Autodesk Inventor part; units mm, degrees
ref_plane "YZ Plane" through (0, 0, 0) normal (1, 0, 0) x (0, 1, 0)
ref_plane "XZ Plane" through (0, 0, 0) normal (0, 1, 0) x (-1, 0, 0)
ref_plane "XY Plane" through (0, 0, 0) normal (0, 0, 1) x (1, 0, 0)
sketch "Esquisse1" plane through (0, 0, 0) normal (0, 1, 0) x (-1, 0, 0)
  circle A0 centre (0, 0) radius 15
  circle A1 centre (0, 0) radius 8
  dimension "d0" = 30
  dimension "d1" = 16
extrude "Extrusion1" add sketch "Esquisse1" along normal blind 5
sketch "Esquisse2" plane through (0, 5, 0) normal (0, 1, 0) x (1, 0, 0)
  circle A0 centre (0, 0) radius 15
  point P0 (-12, 0)
  point P1 (6, -10.3923)
  point P2 (6, 10.3923)
  dimension "d4" = 12
  dimension "d7" = 360
hole "Perçage1" at (-12, 5, 0) at (6, 5, 10.3923) at (6, 5, -10.3923) direction (0, -1, 0) diameter 3 depth 8 tip angle 118
sketch "Esquisse3" plane through (0, 5, 0) normal (0, 1, 0) x (1, 0, 0)
  circle A0 centre (61.032, 0) radius 11
  circle A1 centre (61.032, 0) radius 15
  point P0 (0, 0)
  dimension "d16" = 61.032
  dimension "d17" = 22
  dimension "d18" = 30
extrude "Extrusion2" add sketch "Esquisse3" against normal blind 14
sketch "Esquisse4" plane through (0, 5, 0) normal (0, 1, 0) x (1, 0, 0)
  circle A0 centre (0, 0) radius 8
  line L0 (8, 0) -> (48.6, 0)
  line L1 (48.6, 0) -> (48.6, 2.5)
  line L2 (48.6, 2.5) -> (8, 2.5)
  line L3 (8, 2.5) -> (8, 0)
  line L4 (8, 0) -> (48.6, 0)
  line L5 (48.6, 0) -> (48.6, -2.5)
  line L6 (48.6, -2.5) -> (8, -2.5)
  line L7 (8, -2.5) -> (8, 0)
  dimension "d21" = 2.5
  dimension "d22" = 2.5
  dimension "d23" = 40.6
extrude "Extrusion3" add sketch "Esquisse4" against normal blind 5 contours L3 L2 L1 L0 | L0 L5 L6 L7
properties part number "BarreCodeuseV2"
The model under review builds one solid part; all positions refer to its coordinate system, in mm. A direction names the side the tool comes from. Round coordinates to 2 decimals unless told otherwise and drop trailing zeros. Order: outer loops, then holes, each group sorted by start corner. A loop starts at its lowest first (then second) coordinate and runs counter-clockwise, first axis right, second up.
Item 1: For pin 1 (2.5 mm diameter, centred on x = 6, z = 10.39, fed in from +Y); pin 2 (1 mm diameter, centred on y = -2, z = -10.5, fed in from +X); pin 3 (2 mm diameter, centred on y = -2, z = -7.5, fed in from +X); pin 4 (5.5 mm diameter, centred on x = 30.5, y = 3.5, fed in from -Z), all flat-tipped, find the tip position at first contact; note any pin that passes through.
Working result:
pin 1: passes through
pin 2: stops at x = 72.21
pin 3: stops at x = 74.55
pin 4: stops at z = -2.5
Item 2: To check wall thickness, follow probe 1 along X at (y, z) = (3.85, 0); probe 2 along Z at (x, y) = (0, 2.5); probe 3 along Z at (x, y) = (6, 3.2). State the ranges of each line that lie inside material, in increasing order.
Working result:
probe 1: x = -15 to -13.5, -10.5 to -8, 8 to 50.03, 72.03 to 76.03
probe 2: z = -15 to -8, 8 to 15
probe 3: z = -13.75 to -11.89, -8.89 to -5.29, 5.29 to 8.89, 11.89 to 13.75
Item 3: Add section A-A, the plane x = -12. State the section outline as (y, z) points, and give its area (3 significant figures).
Working result:
outline: (0, -9) - (5, -9) - (5, -1.5) - (0, -1.5) - close; (0, 1.5) - (5, 1.5) - (5, 9) - (0, 9) - close
area: 75.0 mm2
Item 4: Add section B-B, the plane y = 1.5. State the section outline as (x, z) points, and give its area (3 significant figures).
Working result:
outline: (14.79, -2.5) - (46.24, -2.5) arc R15 ccw (long way) to (46.24, 2.5) - (14.79, 2.5) arc R15 ccw (long way) to start; hole circle Ø3 at (-12, 0); hole circle Ø16 at (0, 0); hole circle Ø3 at (6, -10.39); hole circle Ø3 at (6, 10.39); hole circle Ø22 at (61.03, 0)
area: 967 mm2
Item 5: Add section C-C, the plane z = 0. State the section outline as (x, y) points, and give its area (3 significant figures).
Working result:
outline: (-15, 0) - (-13.5, 0) - (-13.5, 5) - (-15, 5) - close; (-10.5, 0) - (-8, 0) - (-8, 5) - (-10.5, 5) - close; (8, 0) - (46.03, 0) - (46.03, -9) - (50.03, -9) - (50.03, 5) - (8, 5) - close; (72.03, -9) - (76.03, -9) - (76.03, 5) - (72.03, 5) - close
area: 322 mm2
Item 6: Machinability: for faces 5 (the flat face through (30, 5, 0)), 6 (the flat face through (9, 0, 0)), which of the approach directions +Z, -Z, +X, -X, +Y, -Y give a long, thin tool a straight path to every point of the face, cutting with its end or side? Answer none if there is none.
Working result:
face 5: +Z, -Z, +X, -X, +Y
face 6: +Z, -Z, -X, -Y
Item 7: Draft analysis for pull direction Z (two halves, no side actions). For faces 1 (the flat face through (31, 3, -2.5)), 2 (the cylindrical face through (-10.536, 2.465, -0.325)), 3 (the cylindrical face through (1.73, 2.46, 7.81)), 4 (the flat face through (31, 3, 2.5)), state which applies: released by +Z, released by -Z, zero draft, split by the parting line, or undercut.
Working result:
face 1: released by -Z
face 2: undercut
face 3: undercut
face 4: released by +Z
Item 8: Add section D-D, the plane x = 6. State the section outline as (y, z) points.
Working result:
outline: (0, -13.75) - (5, -13.75) - (5, -11.89) - (0, -11.89) - close; (0, -8.89) - (5, -8.89) - (5, -5.29) - (0, -5.29) - close; (0, 5.29) - (5, 5.29) - (5, 8.89) - (0, 8.89) - close; (0, 11.89) - (5, 11.89) - (5, 13.75) - (0, 13.75) - close
